Autodesk Inventor part; units mm, degrees
ref_plane "YZ Plane" through (0, 0, 0) normal (1, 0, 0) x (0, 1, 0)
ref_plane "XZ Plane" through (0, 0, 0) normal (0, 1, 0) x (-1, 0, 0)
ref_plane "XY Plane" through (0, 0, 0) normal (0, 0, 1) x (1, 0, 0)
sketch "Sketch12" plane through (0, 0, 0) normal (0, 0, 1) x (1, 0, 0)
  line L0 (37.973, 0) -> (37.973, 12.7)
  line L1 (0, 0) -> (0, 101.6) construction
  line L2 (25.273, 101.6) -> (25.273, 12.7)
  line L3 (25.273, 12.7) -> (37.973, 12.7)
  line L4 (25.273, 101.6) -> (22.733, 101.6)
  line L5 (22.733, 101.6) -> (22.733, 0)
  line L6 (22.733, 0) -> (37.973, 0)
  line L7 (0, -20.32) -> (0, 121.92)
  dimension "d49" = 12.7
  dimension "d50" = 101.6
  dimension "d53" = 2.54
  dimension "d60" = 12.7
  dimension "d72" = 22.733
revolve "Revolution3" add sketch "Sketch12" angle 360 about axis through (0, 0, 0) along (0, 1, 0)
sketch "Sketch13" plane through (0, 0, 0) normal (0, -1, 0) x (1, 0, 0)
  line L0 (0, 0) -> (0, -37.973) construction
  circle A0 centre (0, 0) radius 37.973 construction
  line L1 (0, 0) -> (-3.6396, -37.7982)
  line L2 (0, 0) -> (3.6396, -37.7982)
  arc A1 (-3.6396, -37.7982) -> (3.6396, -37.7982) centre (0, 0) ccw
  dimension "d56" = 5.5
  dimension "d57" = 5.5
extrude "Extrusion5" cut sketch "Sketch13" against normal through all
sketch "Sketch17" plane through (0, 0, 0) normal (0, -1, 0) x (1, 0, 0)
  arc A0 (3.6396, -37.7982) -> (-3.6396, -37.7982) centre (0, 0) ccw
  point P0 (31.75, 0)
  dimension "d73" = 31.75
hole "Hole4" at (31.75, 0, 0) direction (0, 1, 0) diameter 2.6416 end through all counterbore diameter 4.699 counterbore depth 7.1374
pattern_circular "Circular Pattern2" count 6 over 360 about axis through (0, -10, 0) along (0, 1, 0) of "Hole4"
equation "\"d56\" = 0.5 * angleForSlot"
equation "\"d57\" = 0.5 * angleForSlot"
equation "\"angleForSlot\" = 11deg"
properties part number "ExternalStationaryOuterRing" material "LCP Plastic"
Read the model definition and answer for the solid it produces. Units are mm, in the model's axes. A direction names the side the tool comes from. Round coordinates to 2 decimals unless told otherwise and drop trailing zeros. Loops run counter-clockwise (first coordinate to the right, second up) from the corner with the lowest first, then second, coordinate; pieces in that order, holes last.
Q1. Each of these flat-tipped pins is pushed along its axis until it touches: pin 1 (2 mm diameter, centred on y = 20.5, z = 2, fed in from +X); pin 2 (10 mm diameter, centred on x = -2.5, y = 46.5, fed in from +Z); pin 3 (1 mm diameter, centred on x = 12.5, y = 14, fed in from +Z); pin 4 (1 mm diameter, centred on x = -14.5, z = 15, fed in from -Y). Where does it stop, or does it pass through?
Q2. Section A-A on z = 0 is taken. Write down the section's boundary in (x, y), and give its area (3 significant figures).
Q3. Consider probe 1 along X at (y, z) = (11, 0); probe 2 along Y at (x, z) = (-22, 14); probe 3 along X at (y, z) = (32, -15). Determine where each line is inside the solid, lowest interval first.
Q4. Section C-C on z = -14.5 is taken. Write down the section's boundary in (x, y), and give its area (3 significant figures).
Q5. Determine the mould class of faces 3 (the face through (8, 12.7, 25)), 4 (the face through (0.969, 50.089, 22.712)), 5 (the face through (-1.62, 6.44, 37.94)) for opening direction X: released by +X, released by -X, zero draft, split by the parting line, or undercut.
Q6. Section D-D on x = 0 is taken. Write down the section's boundary in (y, z).
Q7. Section B-B on x = 11 is taken. Write down the section's boundary in (y, z), and give its area (3 significant figures).
Q8. Which of the six approach directions +Z, -Z, +X, -X, +Y, -Y give full straight-line access (tool end or side, diameter ignored) to faces 1 (the face through (-23, 101.6, 4)), 2 (the face through (-17.3, 7.137, -27.9))?
Output:
1. pin 1: stops at x = 25.25
1. pin 2: stops at z = 25.27
1. pin 3: stops at z = 22.24
1. pin 4: passes through
2. outline: (-37.97, 0) - (-34.1, 0) - (-34.1, 7.14) - (-33.07, 7.14) - (-33.07, 12.7) - (-37.97, 12.7) - close; (-30.43, 7.14) - (-29.4, 7.14) - (-29.4, 0) - (-22.73, 0) - (-22.73, 101.6) - (-25.27, 101.6) - (-25.27, 12.7) - (-30.43, 12.7) - close; (22.73, 0) - (29.4, 0) - (29.4, 7.14) - (30.43, 7.14) - (30.43, 12.7) - (25.27, 12.7) - (25.27, 101.6) - (22.73, 101.6) - close; (33.07, 7.14) - (34.1, 7.14) - (34.1, 0) - (37.97, 0) - (37.97, 12.7) - (33.07, 12.7) - close
2. area: 742 mm2
3. probe 1: x = -37.97 to -33.07, -30.43 to -22.73, 22.73 to 30.43, 33.07 to 37.97
3. probe 2: y = 0 to 12.7
3. probe 3: x = -20.34 to -17.08, 17.08 to 20.34
4. outline: (-35.1, 0) - (-17.51, 0) - (-17.51, 101.6) - (-20.7, 101.6) - (-20.7, 12.7) - (-35.1, 12.7) - close; (17.51, 0) - (35.1, 0) - (35.1, 12.7) - (20.7, 12.7) - (20.7, 101.6) - (17.51, 101.6) - close
4. area: 1,010 mm2
5. face 3: zero draft
5. face 4: undercut
5. face 5: split by the parting line
6. outline: (0, 22.73) - (101.6, 22.73) - (101.6, 25.27) - (12.7, 25.27) - (12.7, 37.97) - (0, 37.97) - close
7. outline: (0, -36.34) - (12.7, -36.34) - (12.7, -22.75) - (101.6, -22.75) - (101.6, -19.89) - (0, -19.89) - close; (0, 19.89) - (101.6, 19.89) - (101.6, 22.75) - (12.7, 22.75) - (12.7, 36.34) - (0, 36.34) - close
7. area: 926 mm2
8. face 1: +Z, -Z, +X, -X, +Y
8. face 2: -Y
